For this review, use the dimensioned drawing (mm, ordinates from the lowest corner) and the shaded views. Coordinates: 2 decimals unless noted, no trailing zeros. Write each loop counter-clockwise with the first axis right and the second up, starting at its lowest first coordinate (ties: lowest second). Pieces come first, ordered by that corner, then holes. Notation, with made-up numbers: M -18.5,25.5 L -1.5,25.5 A17 cw -1.5,48.5 Z; hole C 41.5,17 d10. An arc over 180 degrees is marked long. Return JSON: item names as keys, results as strings.
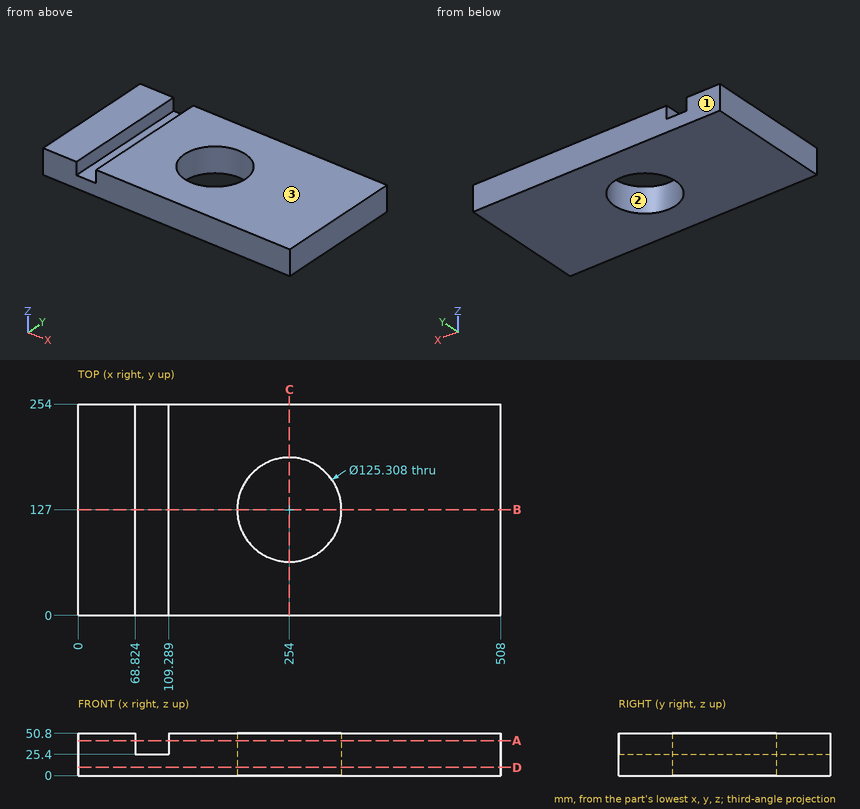
1. Clearance check with flat-ended pins moving along their axes: pin 1 Ø12 at (x, z) = (93, 33.5) entering from +Y; pin 2 Ø6 at (x, z) = (314, 40) entering from -Y. State where each tip first meets the part, or that it passes through.
Checks:
{"pin 1": "through", "pin 2": "y = 0"}
2. Draft analysis for pull direction Y (two halves, no side actions). For the marked faces 1, 2 and 3, state which applies: +Y half, -Y half, draft (parallel to the pull), parting line (faces both ways), or undercut.
Checks:
{"face 1": "+Y half", "face 2": "undercut", "face 3": "draft"}
3. Wall thickness on L1, parallel to Y at x = 254, z = 13; L2, parallel to X at y = 226, z = 32; L3, parallel to X at y = 94.5, z = 27.5 (1 decimal): over which ranges is each line inside the solid? List them lowest first. Write a range as from..to.
Checks:
{"L1": "0..64.35, 189.65..254", "L2": "0..68.82, 109.29..508", "L3": "0..68.8, 109.3..200.4, 307.6..508"}
4. We need section D-D (z = 10). State the section outline as (x, y) points.
Checks:
{"outline": "M 0,0 L 508,0 L 508,254 L 0,254 Z; hole C 254,127 d125.31"}
5. We need section B-B (y = 127). State the section outline as (x, z) points.
Checks:
{"outline": "M 0,0 L 191.35,0 L 191.35,50.8 L 109.29,50.8 L 109.29,25.4 L 68.82,25.4 L 68.82,50.8 L 0,50.8 Z; M 316.65,0 L 508,0 L 508,50.8 L 316.65,50.8 Z"}
6. We need section C-C (x = 254). State the section outline as (y, z) points.
Checks:
{"outline": "M 0,0 L 64.35,0 L 64.35,50.8 L 0,50.8 Z; M 189.65,0 L 254,0 L 254,50.8 L 189.65,50.8 Z"}
7. We need section A-A (z = 42). State the section outline as (x, y) points.
Checks:
{"outline": "M 0,0 L 68.82,0 L 68.82,254 L 0,254 Z; M 109.29,0 L 508,0 L 508,254 L 109.29,254 Z; hole C 254,127 d125.31"}
